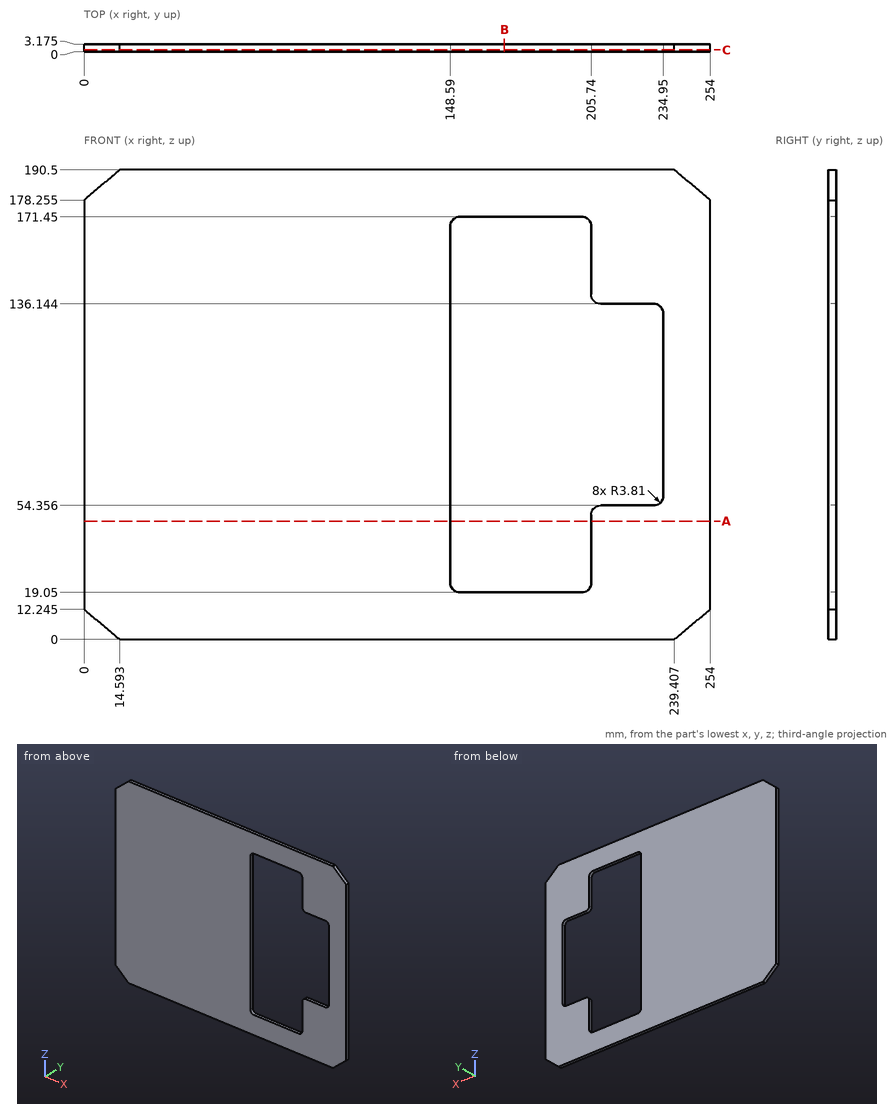
Here's the drawing with two shaded views (mm, measured from the low corner). I have some questions. Round coordinates to 2 decimals unless told otherwise and drop trailing zeros. Order: outer loops, then holes, each group sorted by start corner. A loop starts at its lowest first (then second) coordinate and runs counter-clockwise, first axis right, second up. Notation, with made-up numbers: M 24,25.25 L 73,25.25 A16 ccw 73,41.25 Z; hole C 34,31.5 d10. An arc over 180 degrees is marked long. Use CSV: the item, a comma, the result in double quotes.
1) I need wall thicknesses on line 1 along Z through (x, y) = (211, 0.8); line 2 along X through (y, z) = (2.1, 113); line 3 along X through (y, z) = (2.4, 47). Which ranges of each line are inside material? Lowest first, please. Write a range as [from, to].
Taken from the geometry:
line 1,"[0, 54.36], [136.14, 190.5]"
line 2,"[0, 148.59], [234.95, 254]"
line 3,"[0, 148.59], [205.74, 254]"
2) I want a section at A-A (z = 48). List the corners of the cut face in (x, y) for me (3 decimals), then the cut area to 3 significant figures.
Taken from the geometry:
outline,"M 0,0 L 148.59,0 L 148.59,3.175 L 0,3.175 Z; M 205.74,0 L 254,0 L 254,3.175 L 205.74,3.175 Z"
area,"625 mm^2"
3) I want a section at B-B (x = 170.5). List the corners of the cut face in (y, z) for me (3 decimals), then the cut area to 3 significant figures.
Taken from the geometry:
outline,"M 0,0 L 3.175,0 L 3.175,19.05 L 0,19.05 Z; M 0,171.45 L 3.175,171.45 L 3.175,190.5 L 0,190.5 Z"
area,"121 mm^2"
4) I want a section at C-C (y = 0.75). List the corners of the cut face in (x, z) for me (3 decimals), then the cut area to 3 significant figures.
Taken from the geometry:
outline,"M 0,12.245 L 14.593,0 L 239.407,0 L 254,12.245 L 254,178.255 L 239.407,190.5 L 14.593,190.5 L 0,178.255 Z; hole M 148.59,22.86 A3.81 ccw 152.4,19.05 L 201.93,19.05 A3.81 ccw 205.74,22.86 L 205.74,50.546 A3.81 cw 209.55,54.356 L 231.14,54.356 A3.81 ccw 234.95,58.166 L 234.95,132.334 A3.81 ccw 231.14,136.144 L 209.55,136.144 A3.81 cw 205.74,139.954 L 205.74,167.64 A3.81 ccw 201.93,171.45 L 152.4,171.45 A3.81 ccw 148.59,167.64 Z"
area,"36,900 mm^2"
5) I'm going to push a flat-ended pin straight in: P1, Ø1.6, axis at x = 166.5, y = 2, coming from the -Z side. Where does the tip first touch, or does it pass through?
Taken from the geometry:
P1,"z = 0"
